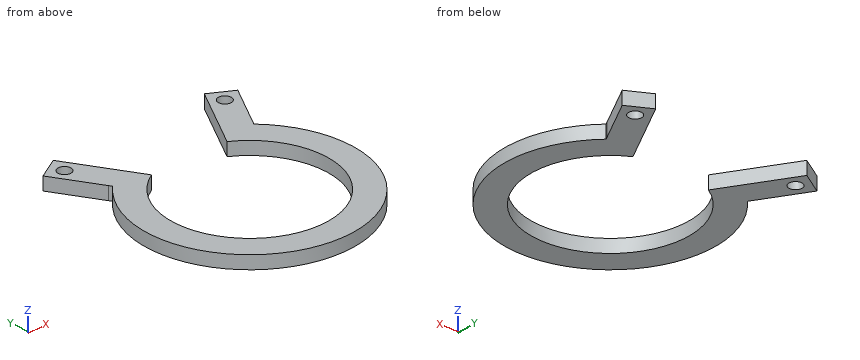
```python
from build123d import *

# Parameters (mm, degrees)
SKETCH2_R           = 25.4
SKETCH2_R_2         = 22.225
SKETCH2_R_3         = 19.05
BOSS_EXTRUDE1_DEPTH = 3.175
SKETCH3_R           = 1.5875
BOSS_EXTRUDE2_DEPTH = 3.175
CUT_EXTRUDE1_DEPTH  = 3.175


with BuildPart() as part:
    # Sketch2 → Boss-Extrude1 (new body)
    with BuildSketch(Plane.XY):
        Circle(SKETCH2_R)
        Circle(SKETCH2_R_2, mode=Mode.SUBTRACT)
        Circle(SKETCH2_R_2)
        Circle(SKETCH2_R_3, mode=Mode.SUBTRACT)
    extrude(amount=BOSS_EXTRUDE1_DEPTH)

    # Sketch3 → Boss-Extrude2 (add)
    with BuildSketch(Plane.XY.offset(3.175)):
        with BuildLine():
            ThreePointArc((-17.795983438, 18.123547486), (-15.370499267, 20.22146761), (-12.7, 21.997045256))
            Line((-12.7, 21.997045256), (-19.05, 32.995567884))
            Line((-19.05, 32.995567884), (-24.549261314, 29.820567884))
            Line((-24.549261314, 29.820567884), (-18.199261314, 18.822045256))
            Line((-18.199261314, 18.822045256), (-17.795983438, 18.123547486))
        make_face()
        with Locations((-20.212130657, 28.658437227)):
            Circle(SKETCH3_R, mode=Mode.SUBTRACT)
        with BuildLine():
            Line((19.05, 32.995567884), (12.7, 21.997045256))
            ThreePointArc((12.7, 21.997045256), (15.370499267, 20.22146761), (17.795983438, 18.123547486))
            Line((17.795983438, 18.123547486), (18.199261314, 18.822045256))
            Line((18.199261314, 18.822045256), (24.549261314, 29.820567884))
            Line((24.549261314, 29.820567884), (19.05, 32.995567884))
        make_face()
        with Locations((20.212130657, 28.658437227)):
            Circle(SKETCH3_R, mode=Mode.SUBTRACT)
    extrude(amount=-BOSS_EXTRUDE2_DEPTH)

    # Sketch5 → Cut-Extrude1 (cut)
    with BuildSketch(Plane.XY.offset(3.175)):
        with BuildLine():
            Line((-12.7, 21.997045256), (0, 0))
            Line((0, 0), (12.7, 21.997045256))
            ThreePointArc((12.7, 21.997045256), (0, 25.4), (-12.7, 21.997045256))
        make_face()
    extrude(amount=-CUT_EXTRUDE1_DEPTH, mode=Mode.SUBTRACT)


solid = part.part
```
Here's how the part is built. I have some questions about the finished solid (model axes, mm). Coordinates: 2 decimals unless noted, no trailing zeros. Write each loop counter-clockwise with the first axis right and the second up, starting at its lowest first coordinate (ties: lowest second). Pieces come first, ordered by that corner, then holes. Notation, with made-up numbers: (-36, 67.5) - (-19, 67.5) arc R15 cw to (-19, 73.5) - close; hole circle Ø8 at (63, -38.75). An arc over 180 degrees is marked (long way). One line per item, written item: value.
1) Suppose I cut it at B-B on y = -3. Write out the boundary of the cut face in (x, z) (3 decimals).
Model answer:
outline: (-25.222, 0) - (-18.812, 0) - (-18.812, 3.175) - (-25.222, 3.175) - close; (18.812, 0) - (25.222, 0) - (25.222, 3.175) - (18.812, 3.175) - close
2) I'm going to push flat-ended pins straight in: P1, Ø1, axis at x = -6.5, z = 1, coming from the +Y side; P2, Ø1.5, axis at y = -2.5, z = 1, coming from the +X side. Where does each tip first touch, or does it pass through?
Model answer:
P1: stops at y = -17.72
P2: stops at x = 25.34
3) I need wall thicknesses on line 1 along X through (y, z) = (0, 1.5); line 2 along Y through (x, z) = (0, 1.95); line 3 along X through (y, z) = (14, 2.5). Which ranges of each line are inside material? Lowest first, please.
Model answer:
line 1: x = -25.4 to -19.05, 19.05 to 25.4
line 2: y = -25.4 to -19.05
line 3: x = -21.19 to -12.92, 12.92 to 21.19
4) Suppose I cut it at C-C on z = 1.8. State how many separate pieces and enclosed holes the cut face has, and give its area (3 significant figures).
Model answer:
separate pieces: 1
enclosed holes: 2
area: 888 mm²
5) Suppose I cut it at A-A on x = 13.5. Write out the boundary of the cut face in (y, z) (3 decimals), and give its area (3 significant figures).
Model answer:
outline: (-21.515, 0) - (-13.441, 0) - (-13.441, 3.175) - (-21.515, 3.175) - close; (13.441, 0) - (23.383, 0) - (23.383, 3.175) - (13.441, 3.175) - close
area: 57.2 mm²
6) Suppose I cut it at D-D on x = 0. Write out the boundary of the cut face in (y, z) (3 decimals).
Model answer:
outline: (-25.4, 0) - (-19.05, 0) - (-19.05, 3.175) - (-25.4, 3.175) - close
